Geometry check sheet. Reference: the model listing, model coordinates, mm. Coordinates: 2 decimals unless noted, no trailing zeros. Write each loop counter-clockwise with the first axis right and the second up, starting at its lowest first coordinate (ties: lowest second). Pieces come first, ordered by that corner, then holes.
from build123d import *

# Parameters (mm, degrees)
SKETCH1_W                                         = 82.55
SKETCH1_H                                         = 25.4
BOSS_EXTRUDE1_DEPTH                               = 1.5875
F_12_0MM_DOWEL_HOLE1_D                            = 12
M3X0_5_TAPPED_HOLE1_D                             = 2.5
CSK_FOR_M2_5_FLAT_HEAD_MACHINE_SCREW1_D           = 2.9
CSK_FOR_M2_5_FLAT_HEAD_MACHINE_SCREW1_CSINK_D     = 5.5
CSK_FOR_M2_5_FLAT_HEAD_MACHINE_SCREW1_CSINK_ANGLE = 90
CUT_EXTRUDE1_DEPTH                                = 44.301226888
FILLET1_R                                         = 1.5875


with BuildPart() as part:
    # Sketch1 → Boss-Extrude1 (new, symmetric)
    with BuildSketch(Plane(origin=(0, 0, 0), x_dir=(1, 0, 0), z_dir=(0, 1, 0))):
        Rectangle(SKETCH1_W, SKETCH1_H)
    extrude(amount=BOSS_EXTRUDE1_DEPTH, both=True)

    # Ø12.0mm Dowel Hole1 (through all)
    with Locations(Plane(origin=(0, 1.5875, 0), x_dir=(1, 0, 0), z_dir=(0, 1, 0))):
        with Locations((0, 0)):
            Hole(F_12_0MM_DOWEL_HOLE1_D / 2)

    # M3x0.5 Tapped Hole1 (through all)
    with Locations(Plane(origin=(0, 1.5875, 0), x_dir=(1, 0, 0), z_dir=(0, 1, 0))):
        with Locations((0, 7.9375), (-7.9375, 0), (7.9375, 0), (0, -7.9375)):
            Hole(M3X0_5_TAPPED_HOLE1_D / 2)

    # CSK for M2.5 Flat Head Machine Screw1 (through all)
    with Locations(Plane(origin=(0, 1.5875, 0), x_dir=(1, 0, 0), z_dir=(0, 1, 0))):
        with Locations((-38.1, 7.9375), (-38.1, -7.9375)):
            csk_for_m2_5_flat_head_machine_screw1 = CounterSinkHole(CSK_FOR_M2_5_FLAT_HEAD_MACHINE_SCREW1_D / 2, CSK_FOR_M2_5_FLAT_HEAD_MACHINE_SCREW1_CSINK_D / 2, counter_sink_angle=CSK_FOR_M2_5_FLAT_HEAD_MACHINE_SCREW1_CSINK_ANGLE)

    # Mirror1: CSK for M2.5 Flat Head Machine Screw1 across plane
    add(csk_for_m2_5_flat_head_machine_screw1.mirror(Plane(origin=(0, 0, 0), x_dir=(0, 0, 1), z_dir=(1, 0, 0))), mode=Mode.SUBTRACT)

    # Sketch14 → Cut-Extrude1 (cut, through all)
    with BuildSketch(Plane(origin=(0, 1.5875, 0), x_dir=(1, 0, 0), z_dir=(0, 1, 0))):
        with BuildLine():
            Line((-33.3375, 7.9375), (-33.3375, -7.9375))
            Line((-33.3375, -7.9375), (-9.461426623, -7.9375))
            ThreePointArc((-9.461426623, -7.9375), (-12.35, 0), (-9.461426623, 7.9375))
            Line((-9.461426623, 7.9375), (-33.3375, 7.9375))
        make_face()
    cut_extrude1 = extrude(amount=-CUT_EXTRUDE1_DEPTH, mode=Mode.SUBTRACT)

    # Mirror2: Cut-Extrude1 across plane
    add(cut_extrude1.mirror(Plane(origin=(0, 0, 0), x_dir=(0, 0, 1), z_dir=(1, 0, 0))), mode=Mode.SUBTRACT)

    # Fillet1
    fillet1_edges = [part.edges().sort_by_distance(p)[0] for p in [
        (-33.3375, 0, -7.9375),
        (-9.461426623, 0, -7.9375),
        (-9.461426623, 0, 7.9375),
        (-33.3375, 0, 7.9375),
        (9.461426623, 0, -7.9375),
        (33.3375, 0, -7.9375),
        (33.3375, 0, 7.9375),
        (9.461426623, 0, 7.9375),
    ]]
    fillet(fillet1_edges, radius=FILLET1_R)


solid = part.part
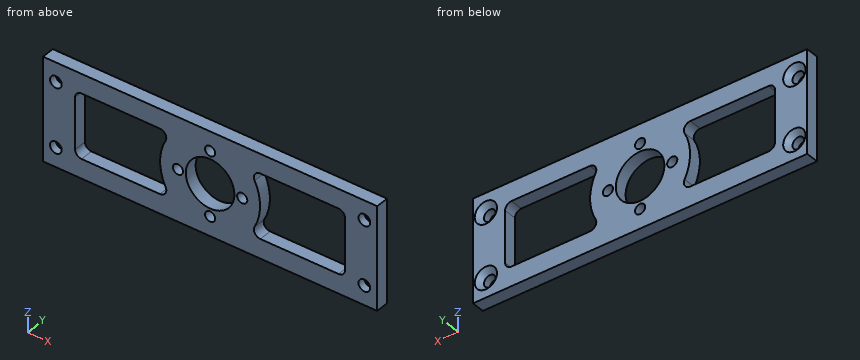
1. Sectioned sample at B-B, the plane z = 0. Give the number of separate pieces and of enclosed holes in the cut face, and give its area (3 significant figures).
Computed values:
separate pieces: 6
enclosed holes: 0
area: 74.9 mm2
2. Sectioned sample at D-D, the plane x = 14.5. Record the boundary of the cut face in (y, z).
Computed values:
outline: (-1.59, -12.7) - (1.59, -12.7) - (1.59, -7.94) - (-1.59, -7.94) - close; (-1.59, 7.94) - (1.59, 7.94) - (1.59, 12.7) - (-1.59, 12.7) - close
3. Sectioned sample at A-A, the plane x = -38.1. Record the boundary of the cut face in (y, z).
Computed values:
outline: (-1.59, -12.7) - (1.59, -12.7) - (1.59, -10.69) - (0.29, -9.39) - (-1.59, -9.39) - close; (-1.59, -6.49) - (0.29, -6.49) - (1.59, -5.19) - (1.59, 5.19) - (0.29, 6.49) - (-1.59, 6.49) - close; (-1.59, 9.39) - (0.29, 9.39) - (1.59, 10.69) - (1.59, 12.7) - (-1.59, 12.7) - close
4. Gauge pin test, flat ends, axial feed: pin 1 Ø1.7 at (x, z) = (-38.1, 7.94) entering from +Y; pin 2 Ø4 at (x, z) = (-38.1, -7.94) entering from +Y; pin 3 Ø3.5 at (x, z) = (38.1, -7.94) entering from +Y. Record the tip position at first contact, or that the pin passes through.
Computed values:
pin 1: passes through
pin 2: stops at y = 0.84
pin 3: stops at y = 0.59
5. Thickness scan on line 1 along X through (y, z) = (-0.5, -8) (3 decimals); line 2 along Z through (x, y) = (-38.1, -0.15); line 3 along Z through (x, y) = (-1, -1.15). Record the ranges inside material, lowest first.
Computed values:
line 1: x = -41.275 to -39.549, -36.651 to -1.248, 1.248 to 36.651, 39.549 to 41.275
line 2: z = -12.7 to -9.39, -6.49 to 6.49, 9.39 to 12.7
line 3: z = -12.7 to -8.69, -7.19 to -5.92, 5.92 to 7.19, 8.69 to 12.7
